Build history of the part. All positions in model axes, mm. A direction names the side the tool comes from. Round coordinates to 2 decimals unless told otherwise and drop trailing zeros. Loops run counter-clockwise (first coordinate to the right, second up) from the corner with the lowest first, then second, coordinate; pieces in that order, holes last. Notation, with made-up numbers: (40.25, 21) - (67.25, 21) arc R29 ccw to (67.25, 59) - close; hole circle Ø1 at (82.25, 22.25). An arc over 180 degrees is marked (long way). Use a Markdown table: item, result.
from build123d import *

# Parameters (mm, degrees)
MODEL_R             = 12.5
MODEL_R_2           = 3
BOSS_EXTRUDE2_DEPTH = 5
FILLET1_R           = 10
FILLET2_R           = 10


with BuildPart() as part:
    # Model → Boss-Extrude2 (new body)
    with BuildSketch(Plane.XY):
        with BuildLine():
            Line((140, 140), (140, 158))
            ThreePointArc((140, 158), (139.414213562, 159.414213562), (138, 160))
            Line((138, 160), (2, 160))
            ThreePointArc((2, 160), (0.585786438, 159.414213562), (0, 158))
            Line((0, 158), (0, 2))
            ThreePointArc((0, 2), (0.585786438, 0.585786438), (2, 0))
            Line((2, 0), (138, 0))
            ThreePointArc((138, 0), (139.414213562, 0.585786438), (140, 2))
            Line((140, 2), (140, 20))
            Line((140, 20), (130, 20))
            ThreePointArc((130, 20), (122.928932188, 17.071067812), (120, 10))
            Line((120, 10), (20, 10))
            ThreePointArc((20, 10), (17.071067812, 17.071067812), (10, 20))
            Line((10, 20), (10, 97))
            Line((10, 97), (61, 97))
            ThreePointArc((61, 97), (62.414213562, 97.585786438), (63, 99))
            Line((63, 99), (63, 150))
            Line((63, 150), (120, 150))
            ThreePointArc((120, 150), (122.928932188, 142.928932188), (130, 140))
            Line((130, 140), (140, 140))
        make_face()
        with Locations((14, 115)):
            Circle(MODEL_R, mode=Mode.SUBTRACT)
        with Locations((45, 115)):
            Circle(MODEL_R, mode=Mode.SUBTRACT)
        with Locations((45, 146)):
            Circle(MODEL_R, mode=Mode.SUBTRACT)
        with Locations((10, 10)):
            Circle(MODEL_R_2, mode=Mode.SUBTRACT)
        with Locations((130, 10)):
            Circle(MODEL_R_2, mode=Mode.SUBTRACT)
        with Locations((130, 150)):
            Circle(MODEL_R_2, mode=Mode.SUBTRACT)
        with Locations((10, 150)):
            Circle(MODEL_R_2, mode=Mode.SUBTRACT)
    extrude(amount=BOSS_EXTRUDE2_DEPTH)

    # Fillet1
    fillet1_edges = [part.edges().sort_by_distance(p)[0] for p in [
        (140, 20, 2.5),
    ]]
    fillet(fillet1_edges, radius=FILLET1_R - 0.0001)  # a hair under: the kernel refuses the full size

    # Fillet2
    fillet2_edges = [part.edges().sort_by_distance(p)[0] for p in [
        (140, 140, 2.5),
    ]]
    fillet(fillet2_edges, radius=FILLET2_R - 0.0001)  # a hair under: the kernel refuses the full size


solid = part.part
Q1. Cut at D-D, the plane x = 45. List the corners of the cut face in (y, z), plus the area to 3 significant figures.
Results found:
| item | result |
|---|---|
| outline | (0, 0) - (10, 0) - (10, 5) - (0, 5) - close; (97, 0) - (102.5, 0) - (102.5, 5) - (97, 5) - close; (127.5, 0) - (133.5, 0) - (133.5, 5) - (127.5, 5) - close; (158.5, 0) - (160, 0) - (160, 5) - (158.5, 5) - close |
| area | 115 mm2 |
Q2. Cut at A-A, the plane x = 117.5. List the corners of the cut face in (y, z).
Results found:
| item | result |
|---|---|
| outline | (0, 0) - (10, 0) - (10, 5) - (0, 5) - close; (150, 0) - (160, 0) - (160, 5) - (150, 5) - close |
Q3. Drop flat-ended pins along their axis: pin 1 (2.5 mm diameter, centred on y = 68.5, z = 3, fed in from +X); pin 2 (3 mm diameter, centred on y = 97, z = 0.5, fed in from +X). Give the stop position or say it passes through.
Results found:
| item | result |
|---|---|
| pin 1 | stops at x = 10 |
| pin 2 | stops at x = 62.94 |
Q4. Which spindle directions (+Z, -Z, +X, -X, +Y, -Y) get a long thin tool onto all of the face, cutting with end or side? Do faces 1 (the face through (69, 0, 2)), 2 (the face through (137.15, 143.01, 2.54)), 3 (the face through (71, 10, 2)). Say none if no direction does.
Results found:
| item | result |
|---|---|
| face 1 | +Z, -Z, +X, -X, -Y |
| face 2 | +Z, -Z, +X |
| face 3 | +Z, -Z |
Q5. Cut at C-C, the plane y = 115. List the corners of the cut face in (x, z).
Results found:
| item | result |
|---|---|
| outline | (0, 0) - (1.5, 0) - (1.5, 5) - (0, 5) - close; (26.5, 0) - (32.5, 0) - (32.5, 5) - (26.5, 5) - close; (57.5, 0) - (63, 0) - (63, 5) - (57.5, 5) - close |
Q6. Pull direction X, two halves, no side cores. Call faces 4 (the face through (10, 58, 2)), 5 (the face through (0, 81, 2)), 6 (the face through (43.373, 127.394, 2.465)): pulls with the +X half, pulls with the -X half, needs draft (parallel to the pull), parting line crosses it, or undercut.
Results found:
| item | result |
|---|---|
| face 4 | pulls with the +X half |
| face 5 | pulls with the -X half |
| face 6 | undercut |
Q7. Cut at B-B, the plane z = 1.45. Count the separate pieces of the cut face and the enclosed holes in it, plus the area to 3 significant figures.
Results found:
| item | result |
|---|---|
| separate pieces | 1 |
| enclosed holes | 7 |
| area | 5,810 mm2 |
Q8. Probe line 1 (Y direction, x = 45, z = 3.45); line 2 (Y direction, x = 88, z = 1.35); line 3 (X direction, y = 110.5, z = 3.1). List the from-to ranges inside material, lowest first.
Results found:
| item | result |
|---|---|
| line 1 | y = 0 to 10, 97 to 102.5, 127.5 to 133.5, 158.5 to 160 |
| line 2 | y = 0 to 10, 150 to 160 |
| line 3 | x = 0 to 2.34, 25.66 to 33.34, 56.66 to 63 |
